Input: part model. Units: mm. Frame: model coordinates. A direction names the side the tool comes from. Round coordinates to 2 decimals unless told otherwise and drop trailing zeros. Loops run counter-clockwise (first coordinate to the right, second up) from the corner with the lowest first, then second, coordinate; pieces in that order, holes last. Notation, with made-up numbers: (27.5, 33) -> (71.5, 33) arc R20 cw to (71.5, 64) -> close; hole circle Ø2 at (59, -10). An arc over 180 degrees is marked (long way). One line per question, with ' | ' between items. Start each with the question number.
Q1. Access query for faces 4 (the face through (1.854, 29, -52)), 5 (the face through (127.31, -0.94, -76.81)). Directions: +Z, -Z, +X, -X, +Y, -Y. A direction counts if a zero-diameter tool reaches every point of the face in a straight line with its end or side. Return the directions, or none.
Q2. Contact query for flat-ended pins moving along their axis: P1, Ø3, axis at y = 27.5, z = -35, coming from the +X side; P2, Ø5, axis at x = 27, z = -14.5, coming from the +Y side. Output: stop coordinate, or through.
Q3. Cut plane B-B on x = 113. Return loops of the section in (y, z), and give its area (3 significant figures).
Q4. Cut plane A-A on z = -43. Return loops of the section in (x, y), and give its area (3 significant figures).
Q5. Cut plane C-C on y = 50.5. Return loops of the section in (x, z).
Q6. Material intervals for L1, parallel to X at y = 7.5, z = -29.5; L2, parallel to Y at x = 104, z = -96, sorted ascending.
Q7. Mould query, pull axis Z, two halves, no side actions, for faces 1 (the face through (1.058, -0.851, -51.511)), 2 (the face through (77, -1, -101.6)), 3 (the face through (68.508, -0.94, -48.425)). Classes: pulls with the +Z half, pulls with the -Z half, needs draft (parallel to the pull), parting line crosses it, or undercut.
from build123d import *

# Parameters (mm, degrees)
SKETCH1_W                    = 152.4
SKETCH1_H                    = 101.6
BASE_FLANGE1_DEPTH           = 1.8542
EDGE_FLANGE1_STRIP_W         = 10.7442
EDGE_FLANGE1_STRIP_H         = 1.8542
EDGE_FLANGE1_STRIP_CUT_DEPTH = 101.6
EDGE_FLANGE1_DEPTH           = 101.6
F_1_4_20_TAPPED_HOLE1_D      = 5.55752
F_3_8_16_TAPPED_HOLE1_D      = 8.1153
F_10_32_TAPPED_HOLE1_D       = 4.3053


# Sheet-metal steps are written as plain solids
with BuildPart() as part:
    # Sketch1 → Base-Flange1 (new body)
    with BuildSketch(Plane(origin=(0, 0, 0), x_dir=(1, 0, 0), z_dir=(0, 1, 0))):
        with Locations((76.2, 50.8)):
            Rectangle(SKETCH1_W, SKETCH1_H)
    extrude(amount=-BASE_FLANGE1_DEPTH)

    # Edge-Flange1 strip (across the edge) → Edge-Flange1 strip cut (cut)
    with BuildSketch(Plane.XY.offset(-101.6)):
        with Locations((-1.8542, -0.9271)):
            Rectangle(EDGE_FLANGE1_STRIP_W, EDGE_FLANGE1_STRIP_H)
    extrude(amount=EDGE_FLANGE1_STRIP_CUT_DEPTH, mode=Mode.SUBTRACT)

    # Edge-Flange1 section (across the edge) → Edge-Flange1 (add)
    with BuildSketch(Plane.XY.offset(-101.6)):
        with BuildLine():
            Line((0, 1.6637), (0, 55.3339))
            Line((0, 55.3339), (1.8542, 55.3339))
            Line((1.8542, 55.3339), (1.8542, 1.6637))
            ThreePointArc((1.8542, 1.6637), (2.341486448, 0.487286448), (3.5179, 0))
            Line((3.5179, 0), (3.5179, -1.8542))
            ThreePointArc((3.5179, -1.8542), (1.030369054, -0.823830946), (0, 1.6637))
        make_face()
    extrude(amount=EDGE_FLANGE1_DEPTH)

    # 1/4-20 Tapped Hole1 (through all)
    with Locations(Plane(origin=(0, 0, 0), x_dir=(1, 0, 0), z_dir=(0, 1, 0))):
        with Locations((129.87815907, 77.870917938), (134.322155935, 26.560738372)):
            Hole(F_1_4_20_TAPPED_HOLE1_D / 2)

    # 3/8-16 Tapped Hole1 (through all)
    with Locations(Plane(origin=(0, 0, 0), x_dir=(1, 0, 0), z_dir=(0, 1, 0))):
        with Locations((70.38044711, 52.025325842)):
            Hole(F_3_8_16_TAPPED_HOLE1_D / 2)

    # #10-32 Tapped Hole1 (through all)
    with Locations(Plane(origin=(6.383092755, 0, -26.580603581), x_dir=(0, 0, 1), z_dir=(0, 1, 0))):
        with Locations((0, 0), (-55.970741812, 0.005307766)):
            Hole(F_10_32_TAPPED_HOLE1_D / 2)


solid = part.part
Results:
1) face 4: +Z, -Z, +X, +Y | face 5: +Y, -Y
2) P1: x = 1.85 | P2: y = 0
3) outline: (-1.85, -101.6) -> (0, -101.6) -> (0, 0) -> (-1.85, 0) -> close | area: 188 mm^2
4) outline: (0, 1.66) arc R3.52 ccw to (3.52, -1.85) -> (152.4, -1.85) -> (152.4, 0) -> (3.52, 0) arc R1.66 cw to (1.85, 1.66) -> (1.85, 55.33) -> (0, 55.33) -> close | area: 383 mm^2
5) outline: (0, -101.6) -> (1.85, -101.6) -> (1.85, 0) -> (0, 0) -> close
6) L1: 0 to 1.85 | L2: -1.85 to 0
7) face 1: needs draft | face 2: pulls with the -Z half | face 3: undercut
